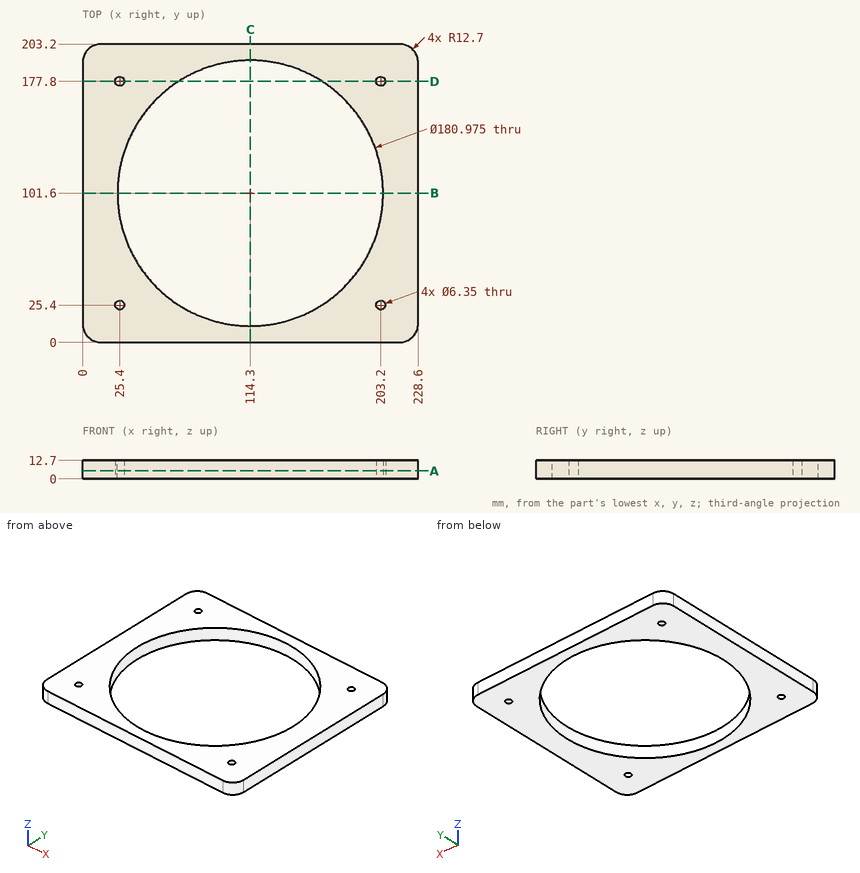
Input: dimensioned drawing with shaded views. Units: mm. Origin: part minimum x, y, z. Round coordinates to 2 decimals unless told otherwise and drop trailing zeros. Order: outer loops, then holes, each group sorted by start corner. A loop starts at its lowest first (then second) coordinate and runs counter-clockwise, first axis right, second up. Notation, with made-up numbers: (67, 88.5) - (94, 88.5) arc R8 ccw to (94, 96.5) - close; hole circle Ø7 at (21.25, 6). An arc over 180 degrees is marked (long way). Write item = value, one per line. Start each with the question number.
Q1. Cut plane C-C on x = 114.3. Return the cut outline in (y, z), and give its area (3 significant figures).
Q2. Cut plane D-D on y = 177.8. Return the cut outline in (x, z) (3 decimals), and give its area (3 significant figures).
Q3. Ray query, line 1 (Y direction, x = 114.3, z = 7); line 2 (X direction, y = 177.8, z = 9.25) (3 decimals); line 3 (Y direction, x = 152, z = 2). Return the intervals inside material, ascending. Write a range as from..to.
Q4. Cut plane B-B on y = 101.6. Return the cut outline in (x, z).
Q5. Cut plane A-A on z = 5.5. Give the number of separate pieces and of enclosed holes in the cut face, and give its area (3 significant figures).
Q6. Pin query (flat end, axial travel): pin 1 (5.5 mm diameter, centred on x = 203.2, y = 25.4, fed in from -Z); pin 2 (1 mm diameter, centred on x = 174.5, y = 176.5, fed in from -Z). Return the tip coordinate at first contact, or that it passes through.
Outcome:
q1.outline = (0, 0) - (11.11, 0) - (11.11, 12.7) - (0, 12.7) - close; (192.09, 0) - (203.2, 0) - (203.2, 12.7) - (192.09, 12.7) - close
q1.area = 282 mm^2
q2.outline = (0, 0) - (22.225, 0) - (22.225, 12.7) - (0, 12.7) - close; (28.575, 0) - (65.499, 0) - (65.499, 12.7) - (28.575, 12.7) - close; (163.101, 0) - (200.025, 0) - (200.025, 12.7) - (163.101, 12.7) - close; (206.375, 0) - (228.6, 0) - (228.6, 12.7) - (206.375, 12.7) - close
q2.area = 1,500 mm^2
q3.line_1 = 0..11.11, 192.09..203.2
q3.line_2 = 0..22.225, 28.575..65.499, 163.101..200.025, 206.375..228.6
q3.line_3 = 0..19.34, 183.86..203.2
q4.outline = (0, 0) - (23.81, 0) - (23.81, 12.7) - (0, 12.7) - close; (204.79, 0) - (228.6, 0) - (228.6, 12.7) - (204.79, 12.7) - close
q5.separate_pieces = 1
q5.enclosed_holes = 5
q5.area = 20,500 mm^2
q6.pin_1 = through
q6.pin_2 = 0
